Input: part model. Units: mm. Frame: model coordinates. Give positions to 0.01 mm unless a question says otherwise; leave off trailing zeros. Write each loop counter-clockwise with the first axis right and the second up, starting at its lowest first coordinate (ties: lowest second). Pieces come first, ordered by that corner, then holes. Notation, with made-up numbers: (-38, 15.5) -> (13, 15.5) arc R19 ccw to (13, 42.5) -> close; hole circle Ø4 at (76, 59). An arc over 180 degrees is marked (long way). Return JSON: item names as keys, results as strings. Group by question number.
Item 1: Section B-B, the plane x = 0. Count the separate pieces of the cut face and the enclosed holes in it, then the cut area to 3 significant figures.
Item 2: Section A-A, the plane y = 1.05. Return loops of the section in (x, z).
Item 3: Line query: line 1 (Z direction, x = -0.5, y = 1.3); line 2 (X direction, y = 1.75, z = -2); line 3 (X direction, y = 1.3, z = 1). Output: solid intervals per line, ascending. Write a range as [from, to].
Item 4: Pin query (flat end, axial travel): P1, Ø5.5, axis at x = -4.98, z = -0.47, coming from the -Y side; P2, Ø4, axis at x = 4.98, z = 0.47, coming from the -Y side; P3, Ø1, axis at x = 2, y = 1.5, coming from the +Z side. Return the tip coordinate at first contact, or that it passes through.
Item 5: Mould query, pull axis Z, two halves, no side actions, for faces 1 (the face through (-6.41, 1.72, -1.39)), 2 (the face through (0, 0, 0)), 3 (the face through (16.855, 0.986, -2.213)). Classes: released by +Z, released by -Z, zero draft, split by the parting line, or undercut.
Item 6: Section D-D, the plane x = -13.5. Return loops of the section in (y, z), then the cut area to 3 significant figures.
from build123d import *

# Parameters (mm, degrees)
SKETCH1_R                                    = 17
BOSS_EXTRUDE1_DEPTH                          = 2
CSK_FOR_M3_COUNTERSUNK_FLAT_HEAD_SCR_2_COUNT = 2
CSK_FOR_M3_COUNTERSUNK_FLAT_HEAD_SCR_2_PITCH = 7.071067812
CSK_FOR_M3_COUNTERSUNK_FLAT_HEAD_SCR_3_COUNT = 2
CSK_FOR_M3_COUNTERSUNK_FLAT_HEAD_SCR_3_PITCH = 10
CSK_FOR_M3_COUNTERSUNK_FLAT_HEAD_SCR_4_COUNT = 2
CSK_FOR_M3_COUNTERSUNK_FLAT_HEAD_SCR_4_PITCH = 7.071067812


with BuildPart() as part:
    # Sketch1 → Boss-Extrude1 (new body)
    with BuildSketch(Plane(origin=(0, 0, 0), x_dir=(1, 0, 0), z_dir=(0, 1, 0))):
        with Locations(Location((0, 0, 0), (0, 0, 270))):
            Circle(SKETCH1_R)
    extrude(amount=BOSS_EXTRUDE1_DEPTH)

    # Sketch3 → CSK for M3 Countersunk Flat Head Screw1 (revolve, cut)
    with BuildSketch(Plane(origin=(-4.977444323, 0, -0.474392252), x_dir=(0, 0, -1), z_dir=(1, 0, 0))):
        Polygon((0, 0), (0, 2), (1.7, 2), (1.7, 1.45), (3.15, 0), align=None)
    csk_for_m3_countersunk_flat_head_screw1 = revolve(axis=Axis((-4.977444323, -6.35, -0.474392252), (0, 1, 0)), mode=Mode.SUBTRACT)

    # CSK for M3 Countersunk Flat Head Scr 2: CSK for M3 Countersunk Flat Head Screw1 ×2
    with Locations(*[Vector(0.7710061224307119, 0, -0.6368277311599726) * (i * CSK_FOR_M3_COUNTERSUNK_FLAT_HEAD_SCR_2_PITCH) for i in range(1, CSK_FOR_M3_COUNTERSUNK_FLAT_HEAD_SCR_2_COUNT)]):
        add(csk_for_m3_countersunk_flat_head_screw1, mode=Mode.SUBTRACT)

    # CSK for M3 Countersunk Flat Head Scr 3: CSK for M3 Countersunk Flat Head Screw1 ×2
    with Locations(*[Vector(0.995488864657962, 0, 0.09487845035624153) * (i * CSK_FOR_M3_COUNTERSUNK_FLAT_HEAD_SCR_3_PITCH) for i in range(1, CSK_FOR_M3_COUNTERSUNK_FLAT_HEAD_SCR_3_COUNT)]):
        add(csk_for_m3_countersunk_flat_head_screw1, mode=Mode.SUBTRACT)

    # CSK for M3 Countersunk Flat Head Scr 4: CSK for M3 Countersunk Flat Head Screw1 ×2
    with Locations(*[Vector(0.6368277311599727, 0, 0.7710061224307118) * (i * CSK_FOR_M3_COUNTERSUNK_FLAT_HEAD_SCR_4_PITCH) for i in range(1, CSK_FOR_M3_COUNTERSUNK_FLAT_HEAD_SCR_4_COUNT)]):
        add(csk_for_m3_countersunk_flat_head_screw1, mode=Mode.SUBTRACT)


solid = part.part
Answer below:
{
 "1": {"separate pieces": "3", "enclosed holes": "0", "area": "50.6 mm2"},
 "2": {"outline": "circle Ø34 at (0, 0); hole circle Ø4.2 at (-4.98, -0.47); hole circle Ø4.2 at (-0.47, 4.98); hole circle Ø4.2 at (0.47, -4.98); hole circle Ø4.2 at (4.98, 0.47)"},
 "3": {"line 1": "z = [-16.99, -6.55], [-3.4, 3.13], [6.83, 16.99]", "line 2": "x = [-16.88, -5.73], [-4.23, 16.88]", "line 3": "x = [-16.97, -6.09], [-3.86, 3.2], [6.75, 16.97]"},
 "4": {"P1": "stops at y = 0.39", "P2": "stops at y = 1.14", "P3": "stops at z = 16.93"},
 "5": {"face 1": "undercut", "face 2": "zero draft", "face 3": "split by the parting line"},
 "6": {"outline": "(0, -10.33) -> (2, -10.33) -> (2, 10.33) -> (0, 10.33) -> close", "area": "41.3 mm2"}
}
